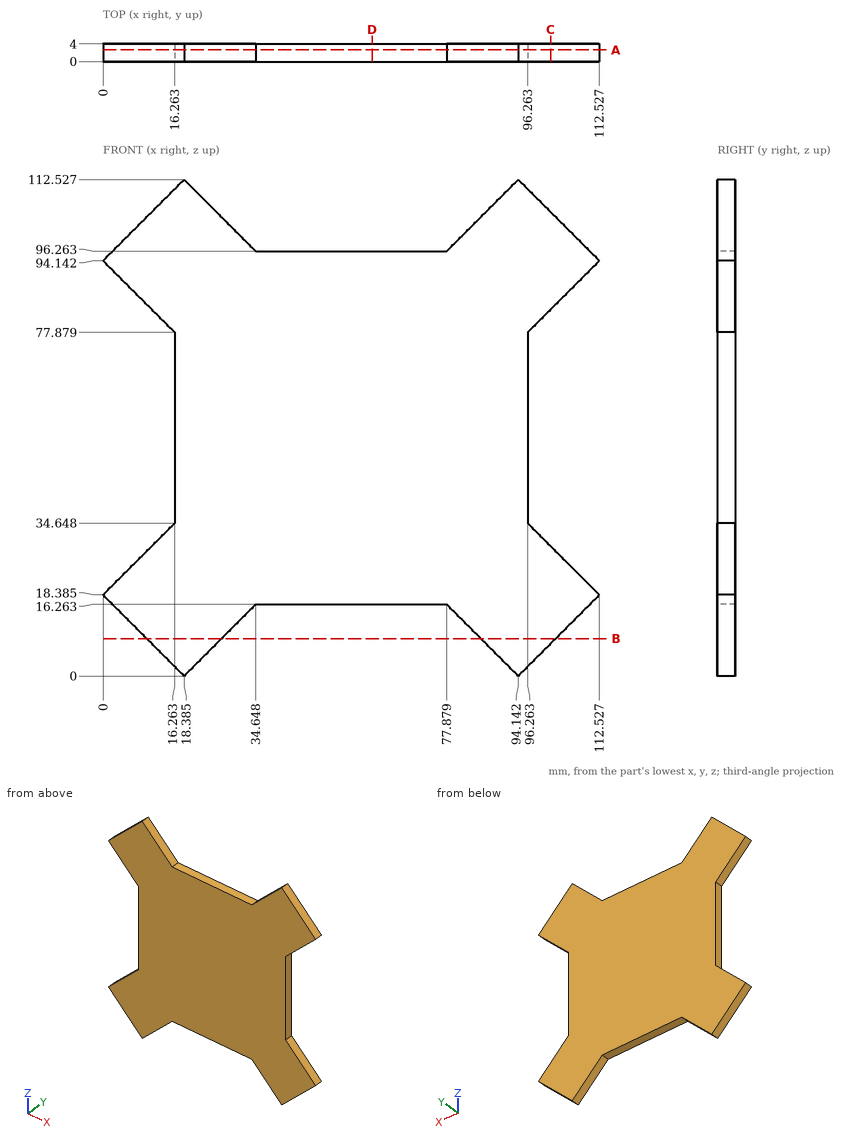
The figure shows three views and two pictorial views of one solid part (mm, origin at its lowest corner). Answer the questions. Coordinates: 2 decimals unless noted, no trailing zeros. Loops run counter-clockwise (first coordinate to the right, second up) from the corner with the lowest first, then second, coordinate; pieces in that order, holes last.
1) Find section C-C on x = 101.5. Write down the section's boundary in (y, z) (1 decimal).
2) Flat-ended cylindrical pins translate along their axes: pin 1 Ø2 at (y, z) = (2, 64) entering from +X; pin 2 Ø2 at (x, y) = (64, 2.5) entering from +Z; pin 3 Ø1.5 at (x, y) = (53.5, 2.5) entering from -Z; pin 4 Ø1 at (x, z) = (38, 69.5) entering from -Y. Find the tip coordinate at first contact, or state that the pin passes through.
3) Find the intervals of material crossed by L1, parallel to Z at x = 57, y = 1.1; L2, parallel to Z at x = 6.5, y = 1.1 (1 decimal), in increasing order.
4) Find section A-A on y = 2.65. Write down the section's boundary in (x, z) (1 decimal).
5) Find section D-D on x = 61. Write down the section's boundary in (y, z).
6) Find section B-B on z = 8.5. Write down the section's boundary in (x, y) (1 decimal).
Values:
1. outline: (0, 7.4) - (4, 7.4) - (4, 29.4) - (0, 29.4) - close; (0, 83.1) - (4, 83.1) - (4, 105.2) - (0, 105.2) - close
2. pin 1: stops at x = 96.26
2. pin 2: stops at z = 96.26
2. pin 3: stops at z = 16.26
2. pin 4: stops at y = 0
3. L1: z = 16.26 to 96.26
3. L2: z = 11.9 to 24.9, 87.6 to 100.6
4. outline: (0, 18.4) - (18.4, 0) - (34.6, 16.3) - (77.9, 16.3) - (94.1, 0) - (112.5, 18.4) - (96.3, 34.6) - (96.3, 77.9) - (112.5, 94.1) - (94.1, 112.5) - (77.9, 96.3) - (34.6, 96.3) - (18.4, 112.5) - (0, 94.1) - (16.3, 77.9) - (16.3, 34.6) - close
5. outline: (0, 16.26) - (4, 16.26) - (4, 96.26) - (0, 96.26) - close
6. outline: (9.9, 0) - (26.9, 0) - (26.9, 4) - (9.9, 4) - close; (85.6, 0) - (102.6, 0) - (102.6, 4) - (85.6, 4) - close
